Check sheet for the modelled part. Datum: model origin and axes. Units: mm. A direction names the side the tool comes from. Round coordinates to 2 decimals unless told otherwise and drop trailing zeros. Order: outer loops, then holes, each group sorted by start corner. A loop starts at its lowest first (then second) coordinate and runs counter-clockwise, first axis right, second up.
Q1. Depth check by flat-ended pin: P1, Ø1.9, axis at y = 3, z = -13, coming from the +X side; P2, Ø1.5, axis at y = 10, z = -17.5, coming from the -X side; P3, Ø2, axis at x = 2.5, y = 7.5, coming from the +Z side. Enter the tip coordinate at first touch or a pass-through.
Q2. Set-up check for faces 4 (the flat face through (12, -1, -2)), 5 (the flat face through (2, 6, -2.6)), 6 (the flat face through (2, 6, -20.4)), 7 (the flat face through (12, -1, -19)), 8 (the flat face through (22, -1, -10)): record each of +Z, -Z, +X, -X, +Y, -Y from which the full face is reachable in a straight line by a thin tool's end or side.
Q3. Cross-section at C-C on y = -1. Record the cut outline in (x, z), then the cut area to 3 significant figures.
Q4. Cross-section at A-A on z = -9.25. Record the cut outline in (x, y), then the cut area to 3 significant figures.
Q5. Cross-section at D-D on z = -17.5. Record the cut outline in (x, y).
Q6. Cross-section at B-B on x = 13. Record the cut outline in (y, z), then the cut area to 3 significant figures.
Q7. Mould release check, pull along X, two halves, no side actions. Record for faces 1 (the flat face through (5.5, 3, -12)), 2 (the flat face through (12.3, 0, -19.3)), 3 (the flat face through (1, 6, -11)): +X half, -X half, draft (parallel to the pull), parting line (faces both ways), or undercut.
Q8. Scan lines: probe 1 along Y at (x, z) = (11.5, -9.5); probe 2 along Z at (x, y) = (7, 2.75); probe 3 along Z at (x, y) = (17.25, -0.5). Record each from-to range of solid material in increasing order.
from build123d import *

# Parameters (mm, degrees)
SKETCH1_W            = 25
SKETCH1_H            = 23
PCB_DEPTH            = 1.6
SIM800L_MODULE_START = 1.6
SKETCH2_W            = 15.8
SKETCH2_H            = 17.8
SIM800L_MODULE_DEPTH = 2.4
HEADER_7PIN_START    = 1.6
SKETCH3_W            = 2.5
SKETCH3_H            = 17.8
HEADER_7PIN_DEPTH    = 8.5
ANTENNA_SPRING_START = 1.6
SKETCH4_R            = 2
ANTENNA_SPRING_DEPTH = 10
SKETCH5_W            = 19
SKETCH5_H            = 17
SIM_HOLDER_DEPTH     = 2


with BuildPart() as part:
    # Sketch1 → PCB (new body)
    with BuildSketch(Plane(origin=(0, 0, 0), x_dir=(1, 0, 0), z_dir=(0, 1, 0))):
        with Locations((12.5, 11.5)):
            Rectangle(SKETCH1_W, SKETCH1_H)
    extrude(amount=PCB_DEPTH)

    # Sketch2 → SIM800L_module (add)
    with BuildSketch(Plane(origin=(0, 0, 0), x_dir=(1, 0, 0), z_dir=(0, 1, 0)).offset(SIM800L_MODULE_START)):
        with Locations((13.4, 11.9)):
            Rectangle(SKETCH2_W, SKETCH2_H)
    extrude(amount=SIM800L_MODULE_DEPTH)

    # Sketch3 → Header_7pin (add)
    with BuildSketch(Plane(origin=(0, 0, 0), x_dir=(1, 0, 0), z_dir=(0, 1, 0)).offset(HEADER_7PIN_START)):
        with Locations((2.25, 11.5)):
            Rectangle(SKETCH3_W, SKETCH3_H)
    extrude(amount=HEADER_7PIN_DEPTH)

    # Sketch4 → Antenna_spring (add)
    with BuildSketch(Plane(origin=(0, 0, 0), x_dir=(1, 0, 0), z_dir=(0, 1, 0)).offset(ANTENNA_SPRING_START)):
        with Locations(Location((22, 19, 0), (0, 0, 115.841932763))):
            Circle(SKETCH4_R)
    extrude(amount=ANTENNA_SPRING_DEPTH)

    # Sketch5 → SIM_holder (add)
    with BuildSketch(Plane(origin=(0, 0, 0), x_dir=(1, 0, 0), z_dir=(0, 1, 0))):
        with Locations((12.5, 10.5)):
            Rectangle(SKETCH5_W, SKETCH5_H)
    extrude(amount=-SIM_HOLDER_DEPTH)


solid = part.part
Results found:
1. P1: stops at x = 21.3
1. P2: stops at x = 1
1. P3: stops at z = -2.6
2. face 4: +Z, +X, -X, -Y
2. face 5: +Z, +X, -X, +Y
2. face 6: -Z, -X, +Y
2. face 7: -Z, +X, -X, -Y
2. face 8: +Z, -Z, +X, -Y
3. outline: (3, -19) - (22, -19) - (22, -2) - (3, -2) - close
3. area: 323 mm2
4. outline: (0, 0) - (3, 0) - (3, -2) - (22, -2) - (22, 0) - (25, 0) - (25, 1.6) - (21.3, 1.6) - (21.3, 4) - (5.5, 4) - (5.5, 1.6) - (3.5, 1.6) - (3.5, 10.1) - (1, 10.1) - (1, 1.6) - (0, 1.6) - close
4. area: 137 mm2
5. outline: (0, 0) - (3, 0) - (3, -2) - (22, -2) - (22, 0) - (25, 0) - (25, 1.6) - (23.32, 1.6) - (23.32, 11.6) - (20.68, 11.6) - (20.68, 4) - (5.5, 4) - (5.5, 1.6) - (3.5, 1.6) - (3.5, 10.1) - (1, 10.1) - (1, 1.6) - (0, 1.6) - close
6. outline: (-2, -19) - (0, -19) - (0, -23) - (1.6, -23) - (1.6, -20.8) - (4, -20.8) - (4, -3) - (1.6, -3) - (1.6, 0) - (0, 0) - (0, -2) - (-2, -2) - close
6. area: 114 mm2
7. face 1: undercut
7. face 2: draft
7. face 3: -X half
8. probe 1: y = -2 to 4
8. probe 2: z = -20.8 to -3
8. probe 3: z = -19 to -2
